from build123d import *

# Parameters (mm, degrees)
F1_DEPTH = 12.7
F2_DEPTH = 9.525


with BuildPart() as f1:
    # F0 (on Front) → F1 (new body)
    with BuildSketch(Plane.XZ):
        Polygon((228.6, 663.575), (88.9, 663.575), (88.9, 644.525), (9.525, 644.525), (9.525, 9.525), (307.975, 9.525), (307.975, 644.525), (228.6, 644.525), align=None)
    extrude(amount=F1_DEPTH)

    # F0 (on Front) → F2 (join)
    with BuildSketch(Plane.XZ):
        Polygon((0, 654.05), (0, 0), (317.5, 0), (317.5, 654.05), (238.125, 654.05), (238.125, 673.1), (79.375, 673.1), (79.375, 654.05), align=None)
        Polygon((88.9, 644.525), (88.9, 663.575), (228.6, 663.575), (228.6, 644.525), (307.975, 644.525), (307.975, 9.525), (9.525, 9.525), (9.525, 644.525), align=None, mode=Mode.SUBTRACT)
    extrude(amount=F2_DEPTH)


solid = f1.part
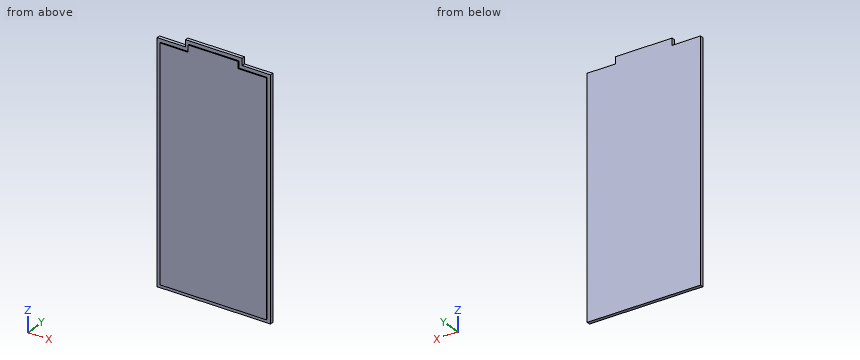
For this review, take the finished solid that the model builds, in its own axes (mm). Round coordinates to 2 decimals unless told otherwise and drop trailing zeros. Loops run counter-clockwise (first coordinate to the right, second up) from the corner with the lowest first, then second, coordinate; pieces in that order, holes last. Notation, with made-up numbers: (-13.75, 49) - (24.25, 49) arc R32 ccw to (24.25, 77) - close; hole circle Ø2 at (33.25, -12.75). An arc over 180 degrees is marked (long way). One line per item, written item: value. Start each with the question number.
Item 1: For L1, parallel to Z at x = 28.5, y = -8.25; L2, parallel to X at y = -11, z = 35 (3 decimals); L3, parallel to Z at x = 221.5, y = -11.5 (3 decimals), list the stretches that pass through material, from the lowest coordinate up.
Item 2: Take a section at B-B (z = 207). Give the boundary of the cut face in (x, y) (3 decimals).
Item 3: Take a section at A-A (x = 291). Give the boundary of the cut face in (y, z) (3 decimals).
Item 4: Clearance check with flat-ended pins moving along their axes: pin 1 Ø5 at (y, z) = (-6.5, 663.5) entering from -X (3 decimals); pin 2 Ø1 at (y, z) = (-11, 290.5) entering from +X (3 decimals); pin 3 Ø3.5 at (x, y) = (230, -12) entering from -Z (3 decimals). State where each tip first meets the part, or that it passes through.
Answer below:
1. L1: z = 0 to 654.05
1. L2: x = 9.525 to 307.975
1. L3: z = 9.525 to 663.575
2. outline: (0, -9.525) - (9.525, -9.525) - (9.525, -12.7) - (307.975, -12.7) - (307.975, -9.525) - (317.5, -9.525) - (317.5, 0) - (0, 0) - close
3. outline: (-12.7, 9.525) - (-9.525, 9.525) - (-9.525, 0) - (0, 0) - (0, 654.05) - (-9.525, 654.05) - (-9.525, 644.525) - (-12.7, 644.525) - close
4. pin 1: stops at x = 79.375
4. pin 2: stops at x = 307.975
4. pin 3: stops at z = 9.525
